Source: CAD feature listing. Evaluate the final solid. Frame: model axes, mm. A direction names the side the tool comes from. Give positions to 0.01 mm unless a question says otherwise; leave off trailing zeros. Order: outer loops, then holes, each group sorted by start corner. A loop starts at its lowest first (then second) coordinate and runs counter-clockwise, first axis right, second up. Notation, with made-up numbers: M 81.5,83.25 L 94.5,83.25 A9 cw 94.5,90.25 Z; hole C -15.75,35.25 d7. An arc over 180 degrees is marked long. Answer in a Markdown table with one row per item. Add a question column.
(1) Set-up query: faces 1 (the face through (9.51, 30.02, -12.98)), 2 (the face through (0, 30, -20.5)). Return all of +Z, -Z, +X, -X, +Y, -Y with unobstructed straight access to the full face (end or side cutting, diameter ignored); none if empty.
(2) Section query B-B, the plane y = 30.95. Return loops of the section in (x, z), plus the area to 3 significant figures.
(3) Section query C-C, the plane z = -12.25. Return loops of the section in (x, y).
(4) Section query D-D, the plane x = 7. Return loops of the section in (y, z).
(5) Pin query (flat end, axial travel): P1, Ø1.5, axis at x = 6.5, z = -1, coming from the +Y side; P2, Ø1, axis at x = -7, y = 29.5, coming from the +Z side; P3, Ø2, axis at x = 0, z = -13.75, coming from the -Y side; P4, Ø1, axis at x = 7.5, y = 30, coming from the +Z side. Return the tip coordinate at first contact, or that it passes through.
(6) Material intervals for line 1 along Z through (x, y) = (0, 30.15); line 2 along Z through (x, y) = (-1, 31.1); line 3 along X through (y, z) = (29.45, -13.75), sorted ascending.
(7) Section query A-A, the plane x = 0. Return loops of the section in (y, z), plus the area to 3 significant figures.
from build123d import *

# Parameters (mm, degrees)
SKETCH006_R                = 1.1
EXTRUDE007_DEPTH           = 3
EXTRUDE007_PLACEMENT_ANGLE = 180
FUSION006_PLACEMENT_ANGLE  = 2
CYLINDER007_R              = 4.1
CYLINDER007_DEPTH          = 3
EXTRUDE005_DEPTH           = 3


with BuildPart() as bearingcoupler_limitswitchmount:
    # Sketch006 → Extrude007 (new body)
    with BuildSketch(Plane.XZ):
        Circle(SKETCH006_R)
        with BuildLine():
            ThreePointArc((-8.4, 0), (-8.259343, -1.53077), (-7.842081, -3.010276))
            ThreePointArc((-9.89596, -3.798682), (-8.474818, -4.431418), (-7.842081, -3.010276))
            ThreePointArc((-10.6, 0), (-10.422504, -1.931687), (-9.89596, -3.798682))
            ThreePointArc((-8.4, 0), (-9.5, 1.1), (-10.6, 0))
        make_face()
    extrude(amount=-EXTRUDE007_DEPTH)


with BuildPart() as bearingcoupler_limitswitchmount_1:
    # Extrude007 placement: moved
    add(bearingcoupler_limitswitchmount.part.rotate(Axis((0, 0, 0), (0, 0, 1)), EXTRUDE007_PLACEMENT_ANGLE))


with BuildPart() as bearingcoupler_limitswitchmount_2:
    # Fusion006 placement: moved
    add(bearingcoupler_limitswitchmount_1.part.moved(Location((0, 0, -13.75))).rotate(Axis((0, 0, -13.75), (0, 1, 0)), FUSION006_PLACEMENT_ANGLE))


with BuildPart() as bearingcoupler_bearinghole:
    # Cylinder007 → Cylinder007 (new body)
    with BuildSketch(Plane.XZ):
        Circle(CYLINDER007_R)
    extrude(amount=CYLINDER007_DEPTH)


with BuildPart() as cut013:
    # Sketch004 → Extrude005 (new body)
    with BuildSketch(Plane(origin=(0, 0, 0), x_dir=(1, 0, 0), z_dir=(0, 1, 0))):
        with BuildLine():
            ThreePointArc((-4.330127, -2.5), (0, -5), (4.330127, -2.5))
            Line((4.330127, -2.5), (5.773503, 0))
            Line((5.773503, 0), (15.33281, 20.5))
            Line((-15.33281, 20.5), (15.33281, 20.5))
            Line((-5.773503, 0), (-15.33281, 20.5))
            Line((-4.330127, -2.5), (-5.773503, 0))
        make_face()
    extrude(amount=-EXTRUDE005_DEPTH)

    # Cut006: cut bearingCoupler_bearingHole
    add(bearingcoupler_bearinghole.part, mode=Mode.SUBTRACT)

    # Cut013: cut bearingCoupler_limitSwitchMount
    add(bearingcoupler_limitswitchmount_2.part, mode=Mode.SUBTRACT)


with BuildPart() as cut013_1:
    # Cut013 placement: moved
    add(cut013.part.moved(Location((0, 31.5, 0))))


solid = cut013_1.part
Values follow:
| question | item | result |
|---|---|---|
| 1 | face 1 | +Y, -Y |
| 1 | face 2 | -Z, +X, -X, +Y, -Y |
| 2 | outline | M -15.33,-20.5 L 15.33,-20.5 L 5.77,0 L 4.33,2.5 A5 ccw -4.33,2.5 L -5.77,0 Z; hole C 0,0 d8.2; hole C 0,-13.75 d2.2; hole M 7.73,-17.03 A1.1 ccw 9.76,-17.89 A10.6 ccw 10.59,-14.12 A1.1 ccw 8.39,-14.04 A8.4 cw Z |
| 2 | area | 405 mm² |
| 3 | outline | M -11.49,28.5 L 11.49,28.5 L 11.49,31.5 L -11.49,31.5 Z |
| 4 | outline | M 28.5,-20.5 L 31.5,-20.5 L 31.5,-2.63 L 28.5,-2.63 Z |
| 5 | P1 | stops at y = 31.5 |
| 5 | P2 | stops at z = -1.56 |
| 5 | P3 | passes through |
| 5 | P4 | stops at z = -2.63 |
| 6 | line 1 | z = -20.5 to -14.85, -12.65 to -4.1, 4.1 to 5 |
| 6 | line 2 | z = -20.5 to -14.21, -13.29 to -3.98, 3.98 to 4.9 |
| 6 | line 3 | x = -12.19 to -1.1, 1.1 to 8.45, 10.54 to 12.19 |
| 7 | outline | M 28.5,-20.5 L 31.5,-20.5 L 31.5,-14.85 L 28.5,-14.85 Z; M 28.5,-12.65 L 31.5,-12.65 L 31.5,-4.1 L 28.5,-4.1 Z; M 28.5,4.1 L 31.5,4.1 L 31.5,5 L 28.5,5 Z |
| 7 | area | 45.3 mm² |
